from build123d import *

# Parameters (mm, degrees)
SKETCH1_R           = 24.651
BOSS_EXTRUDE1_DEPTH = 1
SKETCH12_R          = 10.65
CUT_EXTRUDE11_DEPTH = 10
SKETCH17_R          = 1
CUT_EXTRUDE16_DEPTH = 12


with BuildPart() as part:
    # Sketch1 → Boss-Extrude1 (new body)
    with BuildSketch(Plane(origin=(0, 0, 0), x_dir=(-0.9998860245595664, 0, 0.015097612078282974), z_dir=(0, 1, 0))):
        with BuildLine():
            Line((16.709723735, 8.315025383), (15.933603805, -16.67292447))
            ThreePointArc((15.933603805, -16.67292447), (-46.108257418, -64.086707389), (-105.088045734, -12.914020093))
            Line((-105.088045734, -12.914020093), (-104.311925805, 12.07392976))
            ThreePointArc((-104.311925805, 12.07392976), (-42.270064581, 59.487712679), (16.709723735, 8.315025383))
        make_face()
        with Locations(Location((-44.189161, -2.299497355, 0), (0, 0, 89.134937682))):
            Circle(SKETCH1_R, mode=Mode.SUBTRACT)
    extrude(amount=BOSS_EXTRUDE1_DEPTH)

    # Sketch12 → Cut-Extrude11 (cut)
    with BuildSketch(Plane(origin=(0, 1, 0), x_dir=(1, 0, 0), z_dir=(0, 1, 0))):
        with Locations(Location((68.835159128, -27.448400712, 0), (0, 0, 270))):
            Circle(SKETCH12_R)
        with Locations(Location((18.50605331, -26.645502828, 0), (0, 0, 270))):
            Circle(SKETCH12_R)
        with Locations(Location((10.013422933, 22.180446939, 0), (0, 0, 270))):
            Circle(SKETCH12_R)
        with Locations(Location((78.880907759, 21.081807158, 0), (0, 0, 270))):
            Circle(SKETCH12_R)
    extrude(amount=-CUT_EXTRUDE11_DEPTH, mode=Mode.SUBTRACT)

    # Sketch17 → Cut-Extrude16 (cut)
    with BuildSketch(Plane(origin=(48.22803339, 1, -7.719999561), x_dir=(-0.9998727759206765, 0, -0.01595092388173346), z_dir=(0, 1, 0))):
        with Locations(Location((-7.662813984, 48.486882974, 0), (0, 0, 90.913959377))):
            Circle(SKETCH17_R)
        with Locations(Location((15.667378709, 48.486882974, 0), (0, 0, 90.913959377))):
            Circle(SKETCH17_R)
        with Locations(Location((44.967394337, 23.920411988, 0), (0, 0, 90.913959377))):
            Circle(SKETCH17_R)
        with Locations(Location((49.120943166, 2.107633512, 0), (0, 0, 90.913959377))):
            Circle(SKETCH17_R)
        with Locations(Location((30.899804125, -31.507727626, 0), (0, 0, 90.913959377))):
            Circle(SKETCH17_R)
        with Locations(Location((-22.895239399, -31.507727626, 0), (0, 0, 90.913959377))):
            Circle(SKETCH17_R)
        with Locations(Location((-41.116378441, 2.107633512, 0), (0, 0, 90.913959377))):
            Circle(SKETCH17_R)
        with Locations(Location((-36.962829611, 23.920411988, 0), (0, 0, 90.913959377))):
            Circle(SKETCH17_R)
    extrude(amount=-CUT_EXTRUDE16_DEPTH, mode=Mode.SUBTRACT)


solid = part.part
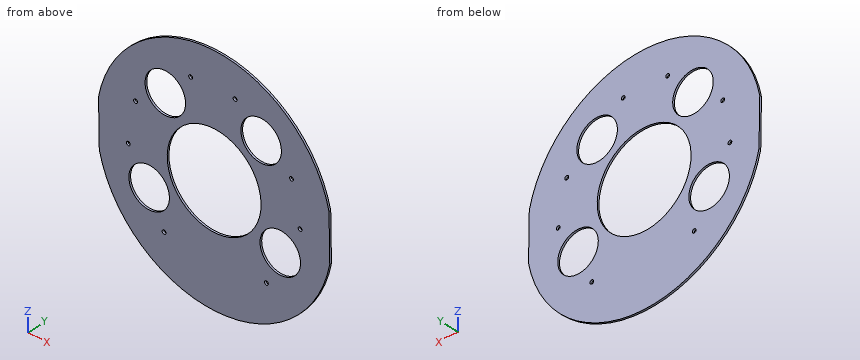
Work out the finished part from the listing and answer in its coordinate system (mm). Round coordinates to 2 decimals unless told otherwise and drop trailing zeros. Write each loop counter-clockwise with the first axis right and the second up, starting at its lowest first coordinate (ties: lowest second). Pieces come first, ordered by that corner, then holes. Notation, with made-up numbers: (58.5, 7.25) - (100.5, 7.25) arc R20 cw to (100.5, 26.25) - close; hole circle Ø4 at (86, -33). An arc over 180 degrees is marked (long way). Answer in a Markdown table with one row per item. Add a question column.
1. Given pin 1 (1.2 mm diameter, centred on x = 55.12, z = 40.88, fed in from +Y); pin 2 (4 mm diameter, centred on x = 81, z = 25.5, fed in from -Y), each flat-ended and moving along its own axis, determine where each tip first touches the part or whether it passes through.
2. Find the intervals of material crossed by line 1 along Z through (x, y) = (10, 0.4); line 2 along Z through (x, y) = (75, 0.25); line 3 along Z through (x, y) = (44, 0.25), in increasing order. Write a range as from..to.
3. A cutting plane is placed at B-B, the plane x = 65.5. Determine the outline of the cut face in (y, z), and give its area (3 significant figures).
4. A cutting plane is placed at D-D, the plane z = -35. Determine the outline of the cut face in (x, y).
5. A cutting plane is placed at C-C, the plane y = 0.45. Count the separate pieces of the cut face and the enclosed holes in it, and give its area (3 significant figures).
6. A cutting plane is placed at A-A, the plane x = 35.5. Determine the outline of the cut face in (y, z).
Worked out:
| question | item | result |
|---|---|---|
| 1 | pin 1 | through |
| 1 | pin 2 | y = 0 |
| 2 | line 1 | -54.49..-32.83, -11.53..20.24, 33.05..48.56 |
| 2 | line 2 | -56.53..-31, -11.16..18.76, 36.13..50.6 |
| 2 | line 3 | -64.78..-27.62, 21.68..58.85 |
| 3 | outline | (0, -60.98) - (1, -60.98) - (1, -15.29) - (0, -15.29) - close; (0, 9.36) - (1, 9.36) - (1, 17.33) - (0, 17.33) - close; (0, 37.56) - (1, 37.56) - (1, 55.05) - (0, 55.05) - close |
| 3 | area | 71.2 mm^2 |
| 4 | outline | (-8.72, 0) - (97.02, 0) - (97.02, 1) - (-8.72, 1) - close |
| 5 | separate pieces | 1 |
| 5 | enclosed holes | 13 |
| 5 | area | 8,600 mm^2 |
| 6 | outline | (0, -64.18) - (1, -64.18) - (1, -26.05) - (0, -26.05) - close; (0, 20.12) - (1, 20.12) - (1, 58.24) - (0, 58.24) - close |
